Can you work these out from the model? Positions are in its coordinate system, mm. Face numbers are marked on the shaded views. A direction names the side the tool comes from. Round coordinates to 2 decimals unless told otherwise and drop trailing zeros. Order: outer loops, then holes, each group sorted by start corner. A loop starts at its lowest first (then second) coordinate and runs counter-clockwise, first axis right, second up. Notation, with made-up numbers: M 57.5,82.25 L 86.5,82.25 A10 ccw 86.5,93.25 Z; hole C -22.5,28 d2. An arc over 180 degrees is marked long. Answer as a JSON object with one key per item and string values. Group by question number.
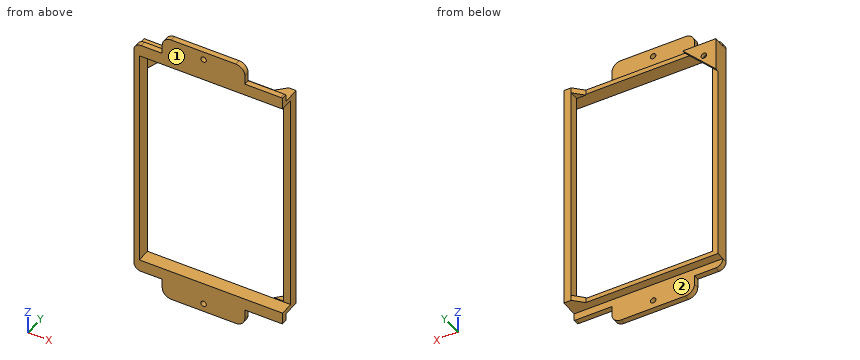
Autodesk Inventor part; units mm, degrees
ref_plane "YZ Plane" through (0, 0, 0) normal (1, 0, 0) x (0, 1, 0)
ref_plane "XZ Plane" through (0, 0, 0) normal (0, 1, 0) x (-1, 0, 0)
ref_plane "XY Plane" through (0, 0, 0) normal (0, 0, 1) x (1, 0, 0)
sketch "Skizze1" plane through (0, 0, 0) normal (0, 1, 0) x (-1, 0, 0)
  line L0 (-39, 60.5) -> (39, 60.5)
  line L1 (39, 60.5) -> (39, -60.5)
  line L2 (39, -60.5) -> (-39, -60.5)
  line L3 (-39, -60.5) -> (-39, 60.5)
  line L4 (-39, 60.5) -> (39, -60.5) construction
  line L5 (39, 60.5) -> (-39, -60.5) construction
  line L6 (42, 63.5) -> (-42, 63.5)
  line L7 (-42, 63.5) -> (-42, -63.5)
  line L8 (-42, -63.5) -> (42, -63.5)
  line L9 (42, -63.5) -> (42, 63.5)
  point P0 (0, 0)
  dimension "d0" = 78
  dimension "d1" = 121
  dimension "d2" = 3
extrude "Extrusion1" add sketch "Skizze1" along normal blind 7.5
sketch "Skizze2" plane through (0, 7.5, 0) normal (0, 1, 0) x (1, 0, 0)
  line L0 (39, -60.5) -> (-39, -60.5)
  line L1 (-39, -60.5) -> (-39, 60.5)
  circle A0 centre (-35.5, -56) radius 1.5
  point P0 (0, 0)
  dimension "d5" = 4.5
  dimension "d6" = 3.5
  dimension "d12" = 3
sketch "Skizze3" plane through (0, 7.5, 0) normal (0, 1, 0) x (1, 0, 0)
  line L0 (-42, -63.5) -> (42, -63.5)
  line L1 (-42, -63.5) -> (-24, -63.5)
  line L2 (-42, -63.5) -> (-42, -45.5)
  line L3 (-42, 63.5) -> (-42, -63.5)
  line L4 (-42, -45.5) -> (-24, -63.5)
  point P0 (0, 0)
  dimension "d7" = 18
  dimension "d9" = 18
extrude "Extrusion2" add sketch "Skizze3" along normal blind 2
extrude "Extrusion3" cut sketch "Skizze2" along normal through all
ref_plane "Arbeitsebene1" through (0, 0, -60.5) normal (1, 0, 0) x (0, 0, -1)
ref_plane "Arbeitsebene2" through (39, 0, 0) normal (0, 0, -1) x (-1, 0, 0)
sketch "Skizze4" plane through (0, 0, 0) normal (0, -1, 0) x (1, 0, 0)
  line L0 (-39, -60.5) -> (-39, 60.5)
  line L1 (-39, 60.5) -> (39, 60.5)
  line L2 (39, 60.5) -> (39, -60.5)
  line L3 (39, -60.5) -> (-39, -60.5)
  line L4 (-42, 63.5) -> (42, 63.5)
  line L5 (-42, -63.5) -> (-42, 63.5)
  line L6 (42, -63.5) -> (-42, -63.5)
  line L7 (42, 63.5) -> (42, -63.5)
  line L8 (-42, 63.5) -> (42, 63.5)
  line L9 (-58.8, 0) -> (58.8, 0) construction
  line L10 (18.5, 63.5) -> (18.5, 72.5)
  line L11 (13.5, 77.5) -> (-21.5, 77.5)
  line L12 (-26.5, 72.5) -> (-26.5, 63.5)
  line L13 (42, 63.5) -> (42, 63.5)
  line L14 (38, 67.5) -> (-38, 67.5)
  line L15 (-42, 63.5) -> (-42, 63.5)
  line L16 (42, -63.5) -> (42, -63.5)
  line L17 (38, -67.5) -> (-38, -67.5)
  line L18 (-42, -63.5) -> (-42, -63.5)
  arc A0 (42, 63.5) -> (38, 67.5) centre (38, 63.5) ccw
  arc A1 (-38, 67.5) -> (-42, 63.5) centre (-38, 63.5) ccw
  arc A2 (-42, -63.5) -> (-38, -67.5) centre (-38, -63.5) ccw
  arc A3 (38, -67.5) -> (42, -63.5) centre (38, -63.5) ccw
  arc A4 (18.5, 72.5) -> (13.5, 77.5) centre (13.5, 72.5) ccw
  arc A5 (-21.5, 77.5) -> (-26.5, 72.5) centre (-21.5, 72.5) ccw
  line L19 (18.5, -63.5) -> (18.5, -72.5)
  line L20 (13.5, -77.5) -> (-21.5, -77.5)
  line L21 (-26.5, -72.5) -> (-26.5, -63.5)
  arc A6 (13.5, -77.5) -> (18.5, -72.5) centre (13.5, -72.5) ccw
  arc A7 (-26.5, -72.5) -> (-21.5, -77.5) centre (-21.5, -72.5) ccw
  line L22 (18.5, -63.5) -> (-26.5, -63.5)
  line L23 (42, -63.5) -> (-42, -63.5)
  line L24 (0, -109.9497) -> (0, 109.9497) construction
  point P0 (0, 0)
  point P1 (18.5, 77.5)
  point P2 (-26.5, 77.5)
  point P3 (-4, 77.5)
  point P4 (42, 67.5)
  point P5 (-42, 67.5)
  point P6 (42, -67.5)
  point P7 (-42, -67.5)
  point P8 (18.5, -77.5)
  point P9 (-26.5, -77.5)
  point P10 (-4, -77.5)
  point P11 (-4, 73)
  point P12 (-4, -73)
  dimension "d20" = 155
  dimension "d21" = 45
  dimension "d22" = 4
  dimension "d23" = 135
  dimension "d24" = 4
  dimension "d25" = 4
  dimension "d26" = 4
  dimension "d27" = 4
  dimension "d30" = 5
  dimension "d33" = 5.5
extrude "Extrusion4" add sketch "Skizze4" against normal blind 3 contours A1 L14 L12 L4 | L12 L14 L10 L4 | L6 L21 L17 A2 | L10 L14 A0 L4 | L6 L19 L17 L21 | L6 A3 L17 L19
extrude "Extrusion5" add sketch "Skizze4" against normal up to surface (3 mm away) contours L12 L14 L10 L4 | L12 A5 L11 A4 L10 L14 | L6 L19 L17 L21 | L17 L19 A6 L20 A7 L21
hole "Bohrung1" at (-4, 0, 73) at (-4, 0, -73) direction (0, 1, 0) diameter 3 end through all
sketch "Skizze6" plane through (42, 7.5, 63.5) normal (1, 0, 0) x (0, 0, -1)
  line L0 (0, -7.5) -> (127, -7.5)
  line L1 (127, -7.5) -> (127, -4.5)
  line L2 (127, -4.5) -> (127, 0)
  line L3 (0, 0) -> (127, 0)
  line L4 (0, -4.5) -> (0, 0)
  line L5 (0, -7.5) -> (0, -4.5)
  line L6 (131, -7.5) -> (127, -7.5)
  line L7 (131, -7.5) -> (131, -4.5)
  line L8 (127, -4.5) -> (131, -4.5)
  line L9 (127, -7.5) -> (127, -4.5)
  line L10 (0, -7.5) -> (-4, -7.5)
  line L11 (0, -7.5) -> (0, -4.5)
  line L12 (-4, -4.5) -> (0, -4.5)
  line L13 (-4, -7.5) -> (-4, -4.5)
  point P0 (63.5, -7.5)
extrude "Extrusion8" cut sketch "Skizze6" against normal up to surface (3 mm away)
sketch "Skizze7" plane through (0, 7.5, 0) normal (0, 1, 0) x (1, 0, 0)
  line L0 (39, -63.5) -> (39, -60.5)
  line L1 (39, -60.5) -> (-27, -60.5)
  line L2 (-27, -60.5) -> (-24, -63.5)
  line L3 (-24, -63.5) -> (39, -63.5)
  line L4 (39, 60.5) -> (39, 63.5)
  line L5 (39, 63.5) -> (-42, 63.5)
  line L6 (-42, 63.5) -> (-42, -45.5)
  line L7 (-42, -45.5) -> (-39, -48.5)
  line L8 (-39, -48.5) -> (-39, 60.5)
  line L9 (-39, 60.5) -> (39, 60.5)
  line L10 (39, -63.5) -> (39, 63.5)
  line L11 (39, 63.5) -> (-42, 63.5)
  line L12 (39, 63.5) -> (35, 63.5)
  line L13 (35, 63.5) -> (35, -63.5)
  line L14 (-42, -63.5) -> (39, -63.5)
  line L15 (35, -63.5) -> (39, -63.5)
  point P0 (0, 0)
  dimension "d48" = 4
extrude "Extrusion9" add sketch "Skizze7" along normal blind 5 contours L3 L13 L1 L0 | L1 L13 L9 L10 | L9 L13 L5 L4
sketch "Skizze8" plane through (-42, 3, -63.5) normal (0, 0, -1) x (-1, 0, 0)
  line L0 (-81, 9.5) -> (-81, 0)
  line L1 (-81, 0) -> (0, 0)
  line L2 (0, 0) -> (0, 4.5)
  line L3 (-77, 4.5) -> (0, 4.5)
  line L4 (-77, 4.5) -> (-77, 9.5)
  line L5 (-81, 9.5) -> (-77, 9.5)
  line L6 (-77, 4.5) -> (-77, 9.5)
  line L7 (-77, 9.5) -> (-72, 4.5)
  line L8 (-77, 4.5) -> (-15, 4.5)
  line L9 (-77, 9.5) -> (-69.9289, 9.5) construction
  line L10 (-72, 4.5) -> (-77, 4.5)
  line L11 (-77, 4.5) -> (-77, 9.5)
  point P0 (-42, -3)
  dimension "d51" = 45
extrude "Extrusion10" add sketch "Skizze8" against normal up to surface (3 mm away) contours L7 L3 L4
sketch "Skizze9" plane through (-42, 9.5, 63.5) normal (0, 0, 1) x (1, 0, 0)
  line L0 (81, -9.5) -> (3, -9.5)
  line L1 (81, -9.5) -> (81, -2)
  line L2 (77, -2) -> (81, -2)
  line L3 (77, 3) -> (77, -2)
  line L4 (77, 3) -> (72, -2)
  line L5 (3, -2) -> (72, -2)
  line L6 (3, -9.5) -> (3, -2)
  line L7 (18, -2) -> (77, -2)
  line L8 (72, -2) -> (77, -2)
  point P0 (42, -9.5)
extrude "Extrusion11" add sketch "Skizze9" against normal up to surface (3 mm away) contours L7 L4 L3
sketch "Skizze10" plane through (0, 0, 0) normal (0, -1, 0) x (1, 0, 0)
  line L0 (39, -67.373) -> (39, -60.5)
  line L1 (39, -60.5) -> (-39, -60.5)
  line L2 (-39, -60.5) -> (-39, 60.5)
  line L3 (-39, 60.5) -> (39, 60.5)
  line L4 (39, 60.5) -> (39, 67.373)
  arc A0 (39, 67.373) -> (38, 67.5) centre (38, 63.5) ccw
  line L5 (38, 67.5) -> (18.5, 67.5)
  line L6 (18.5, 67.5) -> (18.5, 72.5)
  arc A1 (18.5, 72.5) -> (13.5, 77.5) centre (13.5, 72.5) ccw
  line L7 (13.5, 77.5) -> (-21.5, 77.5)
  arc A2 (-21.5, 77.5) -> (-26.5, 72.5) centre (-21.5, 72.5) ccw
  line L8 (-26.5, 72.5) -> (-26.5, 67.5)
  line L9 (-26.5, 67.5) -> (-38, 67.5)
  arc A3 (-38, 67.5) -> (-42, 63.5) centre (-38, 63.5) ccw
  line L10 (-42, -63.5) -> (-42, 63.5)
  arc A4 (-42, -63.5) -> (-38, -67.5) centre (-38, -63.5) ccw
  line L11 (-38, -67.5) -> (-26.5, -67.5)
  line L12 (-26.5, -67.5) -> (-26.5, -72.5)
  arc A5 (-26.5, -72.5) -> (-21.5, -77.5) centre (-21.5, -72.5) ccw
  line L13 (-21.5, -77.5) -> (13.5, -77.5)
  arc A6 (13.5, -77.5) -> (18.5, -72.5) centre (13.5, -72.5) ccw
  line L14 (18.5, -72.5) -> (18.5, -67.5)
  line L15 (18.5, -67.5) -> (38, -67.5)
  arc A7 (38, -67.5) -> (39, -67.373) centre (38, -63.5) ccw
  circle A8 centre (-4, -73) radius 1.5
  circle A9 centre (-4, 73) radius 1.5
  line L16 (39, 61) -> (-39, 61)
  line L17 (-39, -60.5) -> (-39, 60.5)
  line L18 (-39, 60.5) -> (-39, 61)
  line L19 (39, -61) -> (-39, -61)
  line L20 (-39, -61) -> (-39, -60.5)
  point P0 (0, 0)
  dimension "d56" = 0.5
  dimension "d57" = 0.5
extrude "Extrusion12" cut sketch "Skizze10" against normal up to surface (7.5 mm away) contours L19 L20 L1 L0 | L18 L16 L4 L3
properties part number "display_mount"
1) Which directions (+Z, -Z, +X, -X, +Y, -Y) give clear straight access to the entire face, cutting with the end or side of a thin tool? Please do the marked faces 1 and 2.
2) If we section it at C-C on x = -15: Write out the boundary of the cut face in (y, z).
3) For pin 1 (7 mm diameter, centred on x = -13, z = -68, fed in from +Y); pin 2 (3.5 mm diameter, centred on y = 1.5, z = 69, fed in from +X); pin 3 (5 mm diameter, centred on x = 28, z = -56.5, fed in from -Y); pin 4 (2 mm diameter, centred on x = -10.5, z = 63, fed in from +Y), each with a flat end and sliding along its axis, tell me the tip position at first contact or that it passes through.
4) If we section it at A-A on x = -35.5: Write out the boundary of the cut face in (y, z), plus the area to 3 significant figures.
5) If we section it at B-B on y = 11: Write out the boundary of the cut face in (x, z).
6) If we section it at D-D on z = -31: Write out the boundary of the cut face in (x, y).
7) I need wall thicknesses on line 1 along Z through (x, y) = (-4, 2.2); line 2 along X through (y, z) = (0.85, 73); line 3 along Z through (x, y) = (12, 3.75). Which ranges of each line are inside material? Lowest first, please.
Findings:
{
 "1": {"face 1": "+Z, -Z, +X, -X, -Y", "face 2": "-Z, +X, -X, +Y"},
 "2": {"outline": "M 0,-77.5 L 3,-77.5 L 3,-63.5 L 7.5,-63.5 L 7.5,-61 L 0,-61 Z; M 0,61 L 7.5,61 L 7.5,63.5 L 3,63.5 L 3,77.5 L 0,77.5 Z"},
 "3": {"pin 1": "stops at y = 3", "pin 2": "stops at x = 39", "pin 3": "passes through", "pin 4": "stops at y = 7.5"},
 "4": {"outline": "M 0,-67.5 L 3,-67.5 L 3,-63.5 L 7.5,-63.5 L 7.5,-61 L 0,-61 Z; M 0,61 L 7.5,61 L 7.5,57.5 L 9.5,57.5 L 9.5,63.5 L 3,63.5 L 3,67.5 L 0,67.5 Z; M 7.5,52 L 9.5,52 L 9.5,54.5 L 7.5,54.5 Z", "area": "78.5 mm^2"},
 "5": {"outline": "M 33.5,-63.5 L 39,-63.5 L 39,63.5 L 33.5,63.5 L 33.5,60.5 L 35,60.5 L 35,-60.5 L 33.5,-60.5 Z"},
 "6": {"outline": "M -42,0 L -39,0 L -39,7.5 L -42,7.5 Z; M 35,7.5 L 39,7.5 L 39,12.5 L 35,12.5 Z"},
 "7": {"line 1": "z = -77.5 to -74.5, -71.5 to -61, 61 to 71.5, 74.5 to 77.5", "line 2": "x = -26.47 to -5.5, -2.5 to 18.47", "line 3": "z = -63.5 to -61, 61 to 63.5"}
}
